```python
from build123d import *

# Parameters (mm, degrees)
BOSS_EXTRUDE1_DEPTH = 5
SKETCH2_R           = 12.5
SKETCH2_R_2         = 7.5
CUT_EXTRUDE1_DEPTH  = 10


with BuildPart() as part:
    # Sketch1 → Boss-Extrude1 (new body)
    with BuildSketch(Plane(origin=(0, 0, 0), x_dir=(1, 0, 0), z_dir=(0, 1, 0))):
        with BuildLine():
            Line((61.545103008, 13.562628278), (0, 20))
            ThreePointArc((0, 20), (-20, 0), (0, -20))
            Line((0, -20), (2.403061157, -19.855107582))
            Line((2.403061157, -19.855107582), (60.887460049, -16.328794499))
            ThreePointArc((60.887460049, -16.328794499), (74.981046517, -1.685922519), (61.545103008, 13.562628278))
        make_face()
    extrude(amount=BOSS_EXTRUDE1_DEPTH)

    # Sketch2 → Cut-Extrude1 (cut)
    with BuildSketch(Plane(origin=(0, 5, 0), x_dir=(1, 0, 0), z_dir=(0, 1, 0))):
        with Locations(Location((0, 0, 0), (0, 0, 270))):
            Circle(SKETCH2_R)
        with Locations(Location((59.984675549, -1.355986475, 0), (0, 0, 270))):
            Circle(SKETCH2_R_2)
    extrude(amount=-CUT_EXTRUDE1_DEPTH, mode=Mode.SUBTRACT)


solid = part.part
```
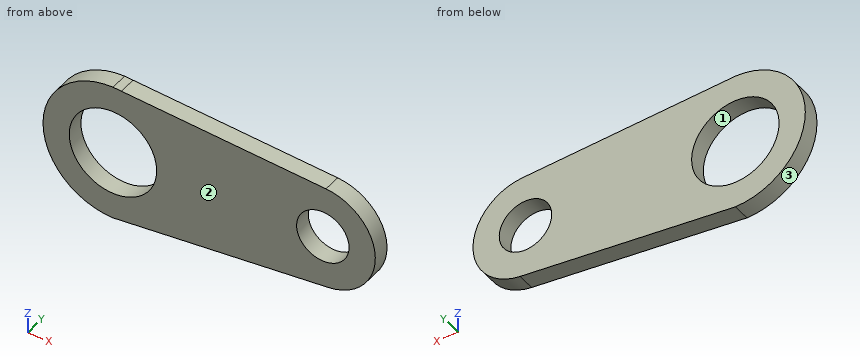
Geometry check sheet. Reference: the model listing, model coordinates, mm. Face numbers are marked on the shaded views. Coordinates: 2 decimals unless noted, no trailing zeros. Loops run counter-clockwise (first coordinate to the right, second up) from the corner with the lowest first, then second, coordinate; pieces in that order, holes last.
Item 1: Sectioned sample at D-D, the plane x = -11. Record the boundary of the cut face in (y, z), then the cut area to 3 significant figures.
Item 2: Go/stop test with flat-tipped pins: pin 1 Ø19.5 at (x, z) = (59.98, 1.36) entering from -Y; pin 2 Ø1 at (x, y) = (16, 3) entering from +Z; pin 3 Ø1 at (y, z) = (1.5, -6) entering from +X. Record where each tip stops, or that it passes through.
Item 3: Sectioned sample at C-C, the plane y = 4.1. Record the boundary of the cut face in (x, z).
Item 4: Sectioned sample at A-A, the plane z = -3. Record the boundary of the cut face in (x, y).
Item 5: Sectioned sample at B-B, the plane x = 64. Record the boundary of the cut face in (y, z).
Item 6: Release check for a two-part mould opening along X. For the marked faces 1, 2 and 3 record: released by +X, released by -X, zero draft, split by the parting line, or undercut.
Item 7: Thickness scan on line 1 (Z direction, x = -0.5, y = 4.4); line 2 (X direction, y = 3, z = -2.5); line 3 (X direction, y = 2, z = 7.5). Record the ranges inside material, lowest first.
Check result:
1. outline: (0, -16.7) - (5, -16.7) - (5, -5.94) - (0, -5.94) - close; (0, 5.94) - (5, 5.94) - (5, 16.7) - (0, 16.7) - close
1. area: 108 mm2
2. pin 1: stops at y = 0
2. pin 2: stops at z = 19.07
2. pin 3: stops at x = 73.33
3. outline: (0, -20) - (61.55, -13.56) arc R15 ccw to (60.89, 16.33) - (0, 20) arc R20 ccw to start; hole circle Ø25 at (0, 0); hole circle Ø15 at (59.98, 1.36)
4. outline: (-19.77, 0) - (-12.13, 0) - (-12.13, 5) - (-19.77, 5) - close; (12.13, 0) - (53.88, 0) - (53.88, 5) - (12.13, 5) - close; (66.09, 0) - (74.34, 0) - (74.34, 5) - (66.09, 5) - close
5. outline: (0, -13.1) - (5, -13.1) - (5, -4.98) - (0, -4.98) - close; (0, 7.69) - (5, 7.69) - (5, 15.81) - (0, 15.81) - close
6. face 1: undercut
6. face 2: zero draft
6. face 3: released by -X
7. line 1: z = -19.99 to -12.49, 12.49 to 19.99
7. line 2: x = -19.84 to -12.25, 12.25 to 53.55, 66.42 to 74.48
7. line 3: x = -18.54 to -10, 10 to 55.68, 64.29 to 73.67
